```python
from build123d import *

# Parameters (mm, degrees)
EXTRUDE_1_DEPTH     = 10
HOLE_WIZARD_M3_1_D  = 2.5
CUT_EXTRUDE_1_DEPTH = 5
FILLET_1_R          = 3


with BuildPart() as part:
    # 草图1 → 凸台-拉伸1 (new body)
    with BuildSketch(Plane(origin=(0, 0, 0), x_dir=(1, 0, 0), z_dir=(0, 1, 0))):
        with BuildLine():
            ThreePointArc((-17.320508076, 10), (-6.840402867, 18.793852416), (6.840402867, 18.793852416))
            Line((6.840402867, 18.793852416), (14.236601546, 25))
            Line((14.236601546, 25), (-8.660254038, 25))
            Line((-8.660254038, 25), (-17.320508076, 10))
        make_face()
        with BuildLine():
            Line((2.136761146, 14.847028383), (6.840402867, 18.793852416))
            ThreePointArc((6.840402867, 18.793852416), (-19.923893962, -1.743114855), (10, -17.320508076))
            Line((10, -17.320508076), (4.682458366, -14.250423982))
            ThreePointArc((4.682458366, -14.250423982), (-14.942920471, -1.307336141), (2.136761146, 14.847028383))
        make_face()
        with BuildLine():
            Line((23.301270189, -25), (10, -17.320508076))
            ThreePointArc((10, -17.320508076), (-5.176380902, -19.318516526), (-17.320508076, -10))
            Line((-17.320508076, -10), (-8.660254038, -25))
            Line((-8.660254038, -25), (23.301270189, -25))
        make_face()
    extrude(amount=EXTRUDE_1_DEPTH)

    # M3 螺纹孔1 (through all)
    with Locations(Plane.XZ):
        with Locations((0, 20), (0, -20)):
            Hole(HOLE_WIZARD_M3_1_D / 2)

    # 草图4 → 切除-拉伸1 (cut)
    with BuildSketch(Plane.XZ):
        with BuildLine():
            Line((0, 15), (-14.43375673, 15))
            Line((-14.43375673, 15), (-17.320508076, 10))
            ThreePointArc((-17.320508076, 10), (-20, 0), (-17.320508076, -10))
            Line((-17.320508076, -10), (-14.43375673, -15))
            Line((-14.43375673, -15), (0, -15))
            Line((0, -15), (0, 15))
        make_face()
    extrude(amount=-CUT_EXTRUDE_1_DEPTH, mode=Mode.SUBTRACT)

    # 圆角1
    fillet_1_edges = [part.edges().sort_by_distance(p)[0] for p in [
        (-8.660254038, 5, -25),
        (14.236601546, 5, -25),
        (2.136761146, 5, -14.847028383),
        (4.682458366, 5, 14.250423982),
        (23.301270189, 5, 25),
        (-8.660254038, 5, 25),
        (-14.43375673, 2.5, -15),
        (-14.43375673, 2.5, 15),
    ]]
    fillet(fillet_1_edges, radius=FILLET_1_R)


solid = part.part
```
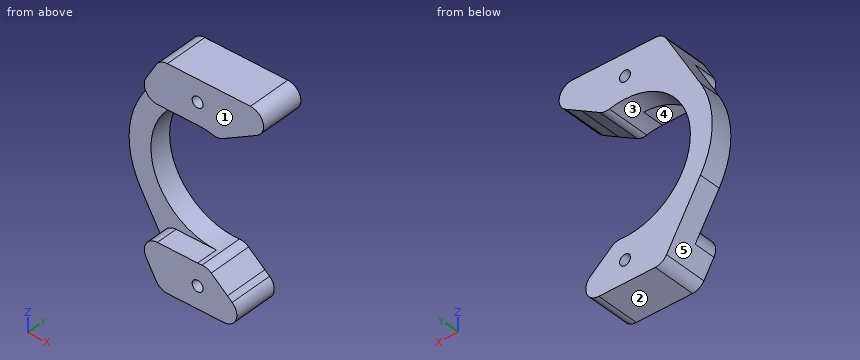
Verification items for the finished model (mm, model axes). Face numbers are marked on the shaded views. A direction names the side the tool comes from. Coordinates: 2 decimals unless noted, no trailing zeros. Loops run counter-clockwise (first coordinate to the right, second up) from the corner with the lowest first, then second, coordinate; pieces in that order, holes last. Notation, with made-up numbers: (76, 76.5) -> (106, 76.5) arc R22 cw to (106, 84.5) -> close; hole circle Ø2 at (39, 48.5). An arc over 180 degrees is marked (long way). Answer in a Markdown table with one row per item. Add a question column.
1. Section check B-B, the plane x = -7.5. Enter the section's corners in (y, z) (3 decimals).
2. Section check D-D, the plane z = -17. Enter the section's corners in (x, y), then the cut area to 3 significant figures.
3. Material ranges on probe 1 along Z at (x, y) = (0, 2); probe 2 along Z at (x, y) = (-1, 7.5); probe 3 along Z at (x, y) = (10, 5.5), recorded low to high. Write a range as [from, to].
4. Access from +Z, -Z, +X, -X, +Y, -Y to the whole of each face (thin tool, end or side, straight path). Record for the marked faces 4 and 5.
5. Section check C-C, the plane z = 20. Enter the section's corners in (x, y).
6. Depth check by flat-ended pin: P1, Ø10, axis at x = -5, z = 9.5, coming from the -Y side; P2, Ø1.5, axis at x = 0, z = 20, coming from the -Y side; P3, Ø1, axis at y = 5, z = 5.5, coming from the -X side. Enter the tip coordinate at first touch or a pass-through.
7. Section check A-A, the plane y = 2.5. Enter the section's corners in (x, z).
8. Draft check along Z on the marked faces 1, 2 and 3. Enter one of: +Z half, -Z half, draft (parallel to the pull), parting line (faces both ways), or undercut.
Derived:
| question | item | result |
|---|---|---|
| 1 | outline | (0, -24.945) -> (10, -24.945) -> (10, -12.99) -> (5, -12.99) -> (5, -15) -> (0, -15) -> close; (0, 15) -> (5, 15) -> (5, 12.99) -> (10, 12.99) -> (10, 24.945) -> (0, 24.945) -> close |
| 2 | outline | (-13.28, 5) -> (-12.07, 5) -> (-12.07, 0) -> (4.7, 0) -> (4.7, 10) -> (-13.28, 10) -> close |
| 2 | area | 174 mm² |
| 3 | probe 1 | z = [-25, -21.25], [-18.75, -15], [15, 18.75], [21.25, 25] |
| 3 | probe 2 | z = [-25, -20.75], [-19.25, -14.97], [14.97, 19.25], [20.75, 25] |
| 3 | probe 3 | z = [17.32, 25] |
| 4 | face 4 | -X, -Y |
| 4 | face 5 | -Z, -X, +Y, -Y |
| 5 | outline | (-11.55, 0) -> (-1.25, 0) -> (-1.25, 10) -> (-11.55, 10) -> close; (1.25, 0) -> (14.34, 0) -> (14.34, 10) -> (1.25, 10) -> close |
| 6 | P1 | stops at y = 5 |
| 6 | P2 | passes through |
| 6 | P3 | stops at x = -19.36 |
| 7 | outline | (-11.84, -19.5) -> (-9.53, -23.5) arc R3 ccw to (-6.93, -25) -> (5.99, -25) arc R3 ccw to (7.92, -19.7) -> (3.11, -15.66) arc R3 ccw to (0.98, -14.97) arc R15 cw to (0, -15) -> (-9.24, -15) arc R3 ccw to start; (-11.84, 19.5) arc R3 ccw to (-9.24, 15) -> (0, 15) arc R15 cw to (3.57, 14.57) arc R3 ccw to (5.78, 14.89) -> (13.61, 19.4) arc R3 ccw to (12.11, 25) -> (-6.93, 25) arc R3 ccw to (-9.53, 23.5) -> close; hole circle Ø2.5 at (0, -20); hole circle Ø2.5 at (0, 20) |
| 8 | face 1 | draft |
| 8 | face 2 | -Z half |
| 8 | face 3 | undercut |
